```python
from build123d import *

# Parameters (mm, degrees)
BOSS_EXTRUDE1_DEPTH                             = 40
SKETCH4_R                                       = 23
CUT_EXTRUDE1_DEPTH                              = 15
BOSS_EXTRUDE3_DEPTH                             = 20
CSK_FOR_M2_OVAL_HEAD_MACHINE_SCREW1_D           = 43
CSK_FOR_M2_OVAL_HEAD_MACHINE_SCREW1_CSINK_D     = 53
CSK_FOR_M2_OVAL_HEAD_MACHINE_SCREW1_CSINK_ANGLE = 90
SKETCH18_W                                      = 15
SKETCH18_H                                      = 25
M2_CLEARANCE_HOLE1_AT_2_COUNT                   = 2
M2_CLEARANCE_HOLE1_AT_2_PITCH                   = 135
M2_CLEARANCE_HOLE1_AT_3_COUNT                   = 2
M2_CLEARANCE_HOLE1_AT_3_PITCH                   = 135


with BuildPart() as part:
    # Sketch1 → Boss-Extrude1 (new body)
    with BuildSketch(Plane(origin=(0, 0, 0), x_dir=(1, 0, 0), z_dir=(0, 1, 0))):
        with BuildLine():
            Line((64.951905284, 0), (199.951905284, 0))
            ThreePointArc((199.951905284, 0), (232.427857926, 18.75), (232.427857926, 56.25))
            Line((232.427857926, 56.25), (164.927857926, 173.163429511))
            ThreePointArc((164.927857926, 173.163429511), (132.451905284, 191.913429511), (99.975952642, 173.163429511))
            Line((99.975952642, 173.163429511), (32.475952642, 56.25))
            ThreePointArc((32.475952642, 56.25), (32.475952642, 18.75), (64.951905284, 0))
        make_face()
    extrude(amount=BOSS_EXTRUDE1_DEPTH)

    # Sketch4 → Cut-Extrude1 (cut)
    with BuildSketch(Plane(origin=(0, 40, 0), x_dir=(1, 0, 0), z_dir=(0, 1, 0))):
        with Locations(Location((64.951905284, 37.5, 0), (0, 0, 270))):
            Circle(SKETCH4_R)
        with Locations(Location((199.951905284, 37.5, 0), (0, 0, 270))):
            Circle(SKETCH4_R)
        with Locations(Location((132.451905284, 154.413429511, 0), (0, 0, 270))):
            Circle(SKETCH4_R)
    extrude(amount=-CUT_EXTRUDE1_DEPTH, mode=Mode.SUBTRACT)

    # Sketch16 → Boss-Extrude3 (add, symmetric)
    with BuildSketch(Plane(origin=(132.451905284, 0, 0), x_dir=(0, 0, -1), z_dir=(1, 0, 0))):
        with BuildLine():
            Line((-120.086570489, 0), (0, 0))
            Line((0, 0), (37.5, 0))
            Line((37.5, 0), (37.5, 40))
            ThreePointArc((37.5, 40), (-27.641071176, 54.533483722), (-83.385649061, 91.236662594))
            ThreePointArc((-83.385649061, 91.236662594), (-169.257411022, 72.779495475), (-120.086570489, 0))
        make_face()
    extrude(amount=BOSS_EXTRUDE3_DEPTH, both=True)

    # CSK for M2 Oval Head Machine Screw1 (through all)
    with Locations(Plane(origin=(152.451905284, 53, 120.086570489), x_dir=(0, 0, 1), z_dir=(1, 0, 0))):
        with Locations((0, 0)):
            CounterSinkHole(CSK_FOR_M2_OVAL_HEAD_MACHINE_SCREW1_D / 2, CSK_FOR_M2_OVAL_HEAD_MACHINE_SCREW1_CSINK_D / 2, counter_sink_angle=CSK_FOR_M2_OVAL_HEAD_MACHINE_SCREW1_CSINK_ANGLE)

    # Sketch18 → M2 Clearance Hole1 (revolve, cut)
    with BuildSketch(Plane(origin=(64.951905284, 25, -37.5), x_dir=(0, 0, 1), z_dir=(1, 0, 0))):
        with Locations((7.5, 12.5)):
            Rectangle(SKETCH18_W, SKETCH18_H)
    m2_clearance_hole1 = revolve(axis=Axis((64.951905284, 31.35, -37.5), (0, -1, 0)), mode=Mode.SUBTRACT)

    # M2 Clearance Hole1 at 2: M2 Clearance Hole1 ×2
    with Locations(*[(i * M2_CLEARANCE_HOLE1_AT_2_PITCH, 0, 0) for i in range(1, M2_CLEARANCE_HOLE1_AT_2_COUNT)]):
        add(m2_clearance_hole1, mode=Mode.SUBTRACT)

    # M2 Clearance Hole1 at 3: M2 Clearance Hole1 ×2
    with Locations(*[Vector(0.49999999999999206, 0, -0.8660254037844433) * (i * M2_CLEARANCE_HOLE1_AT_3_PITCH) for i in range(1, M2_CLEARANCE_HOLE1_AT_3_COUNT)]):
        add(m2_clearance_hole1, mode=Mode.SUBTRACT)


solid = part.part
```
Source: CAD feature listing. Evaluate the final solid. Frame: model axes, mm. A direction names the side the tool comes from. Round coordinates to 2 decimals unless told otherwise and drop trailing zeros. Loops run counter-clockwise (first coordinate to the right, second up) from the corner with the lowest first, then second, coordinate; pieces in that order, holes last. Notation, with made-up numbers: (1, 8.25) - (16, 8.25) arc R20 ccw to (16, 39.25) - close; hole circle Ø1 at (6, 41). An arc over 180 degrees is marked (long way). Use CSV: the item, a comma, the result in double quotes.
Q1. Mould query, pull axis X, two halves, no side actions, for faces 4 (the cylindrical face through (132.73, 54.17, 26.78)), 5 (the flat face through (199.15, 19.72, -113.89)), 6 (the flat face through (65, 25, -22)), 7 (the flat face through (112.452, 42, 93)). Classes: pulls with the +X half, pulls with the -X half, needs draft (parallel to the pull), parting line crosses it, or undercut.
Reported:
face 4,"needs draft"
face 5,"pulls with the +X half"
face 6,"undercut"
face 7,"pulls with the -X half"
Q2. Section query C-C, the plane z = 21. Output: boundary loops of the cut face in (x, y), then the cut area to 3 significant figures.
Reported:
outline,"(112.45, 0) - (152.45, 0) - (152.45, 51.87) - (112.45, 51.87) - close"
area,"2,070 mm^2"
Q3. Section query D-D, the plane y = 97.5. Output: boundary loops of the cut face in (x, z), then the cut area to 3 significant figures.
Reported:
outline,"(112.45, 91.3) - (152.45, 91.3) - (152.45, 148.87) - (112.45, 148.87) - close"
area,"2,300 mm^2"
Q4. Section query A-A, the plane x = 141. Output: boundary loops of the cut face in (y, z), then the cut area to 3 significant figures.
Reported:
outline,"(0, -190.93) - (40, -190.93) - (40, -175.77) - (25, -175.77) - (25, -166.74) - (0, -166.74) - close; (0, -142.09) - (25, -142.09) - (25, -133.06) - (40, -133.06) - (40, -37.5) arc R185 cw to (91.24, 83.39) arc R53 ccw (long way) to (0, 120.09) - close; hole circle Ø43 at (53, 120.09)"
area,"18,400 mm^2"
Q5. Ray query, line 1 along X through (y, z) = (35, -37); line 2 along X through (y, z) = (5, -37.5); line 3 along Y through (x, z) = (120.5, -72.5). Return the intervals inside material, ascending.
Reported:
line 1,"27.46 to 41.96, 87.95 to 176.96, 222.95 to 237.45"
line 2,"27.45 to 49.95, 79.95 to 184.95, 214.95 to 237.45"
line 3,"0 to 40"
Q6. Pin query (flat end, axial travel): pin 1 Ø10 at (y, z) = (31, 50.5) entering from -X; pin 2 Ø23 at (x, z) = (132.5, -148) entering from +Y; pin 3 Ø12 at (x, y) = (123.5, 94.5) entering from -Z; pin 4 Ø10 at (y, z) = (45.5, -36.5) entering from +X. Return the tip coordinate at first contact, or that it passes through.
Reported:
pin 1,"x = 112.45"
pin 2,"y = 25"
pin 3,"z = 80.46"
pin 4,"through"
Q7. Section query B-B, the plane y = 53. Output: boundary loops of the cut face in (x, z), then the cut area to 3 significant figures.
Reported:
outline,"(112.45, 23.91) - (152.45, 23.91) - (152.45, 93.59) - (147.45, 98.59) - (112.45, 98.59) - close; (112.45, 141.59) - (147.45, 141.59) - (152.45, 146.59) - (152.45, 173.09) - (112.45, 173.09) - close"
area,"4,220 mm^2"
Q8. Reachability of faces 1 (the flat face through (88, 20, 0)), 2 (the cylindrical face through (44.547, 32.605, -26.887)), 3 (the flat face through (66.7, 19.72, -115.53)) from +Z, -Z, +X, -X, +Y, -Y: full face, straight path, thin tool, end or side. Return the list, or none.
Reported:
face 1,"+Z, -X, +Y, -Y"
face 2,"+Y"
face 3,"-Z, -X, +Y, -Y"
